Source: three-view drawing plus pictorial views. Frame: mm from the lowest corner of the part. Give positions to 0.01 mm unless a question says otherwise; leave off trailing zeros. Loops run counter-clockwise (first coordinate to the right, second up) from the corner with the lowest first, then second, coordinate; pieces in that order, holes last. Notation, with made-up numbers: (54.25, -36) - (74.25, -36) arc R22 ccw to (74.25, 2) - close; hole circle Ø5 at (47, -17.5). An arc over 180 degrees is marked (long way). Answer as a JSON object with one key per item and string values.
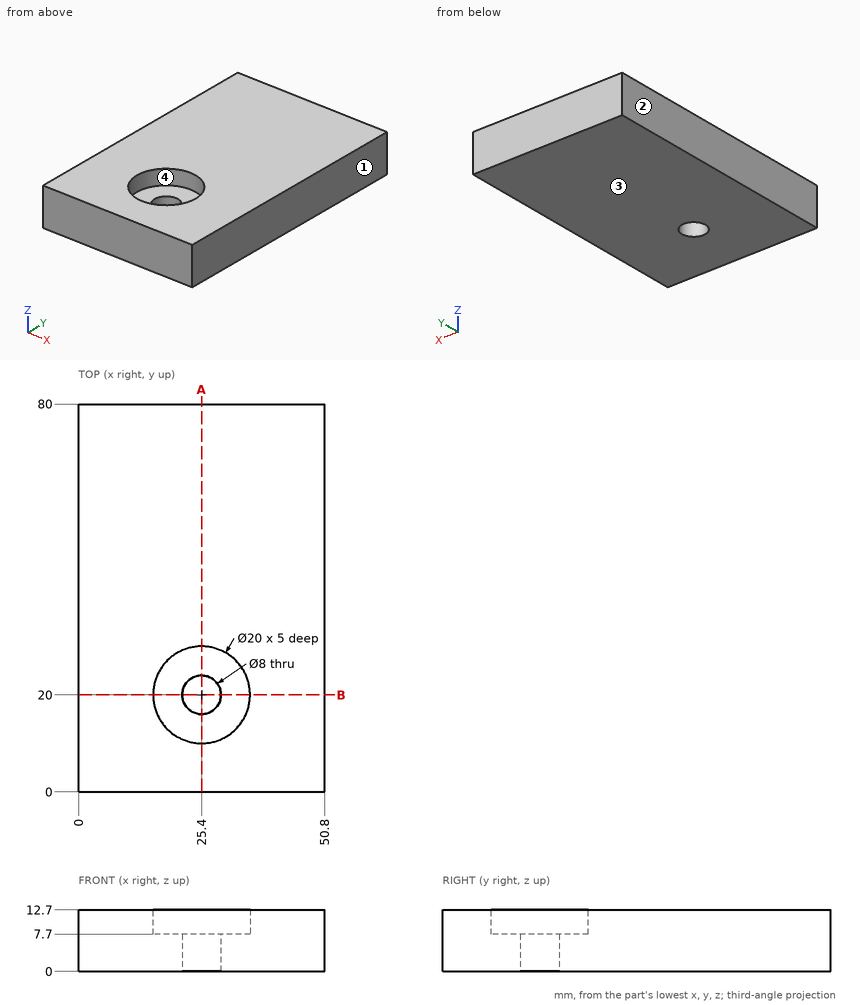
Item 1: Cut plane B-B (y = 20). Return loops of the section in (x, z).
Geometry check:
{"outline": "(0, 0) - (21.4, 0) - (21.4, 7.7) - (15.4, 7.7) - (15.4, 12.7) - (0, 12.7) - close; (29.4, 0) - (50.8, 0) - (50.8, 12.7) - (35.4, 12.7) - (35.4, 7.7) - (29.4, 7.7) - close"}
Item 2: Contact query for a flat-ended pin moving along its axis: P1, Ø12, axis at x = 25.4, y = 20, coming from the +Z side. Output: stop coordinate, or through.
Geometry check:
{"P1": "stops at z = 7.7"}
Item 3: Cut plane A-A (x = 25.4). Return loops of the section in (y, z).
Geometry check:
{"outline": "(0, 0) - (16, 0) - (16, 7.7) - (10, 7.7) - (10, 12.7) - (0, 12.7) - close; (24, 0) - (80, 0) - (80, 12.7) - (30, 12.7) - (30, 7.7) - (24, 7.7) - close"}
Item 4: Material intervals for line 1 (X direction, y = 20, z = 5); line 2 (Y direction, x = 25.4, z = 9.75); line 3 (Y direction, x = 25.4, z = 2.75), sorted ascending. Write a range as [from, to].
Geometry check:
{"line 1": "x = [0, 21.4], [29.4, 50.8]", "line 2": "y = [0, 10], [30, 80]", "line 3": "y = [0, 16], [24, 80]"}
Item 5: Mould query, pull axis X, two halves, no side actions, for the marked faces 1, 2, 3 and 4. Classes: released by +X, released by -X, zero draft, split by the parting line, or undercut.
Geometry check:
{"face 1": "released by +X", "face 2": "released by -X", "face 3": "zero draft", "face 4": "undercut"}
